Build history of the part. All positions in model axes, mm. Round coordinates to 2 decimals unless told otherwise and drop trailing zeros. Order: outer loops, then holes, each group sorted by start corner. A loop starts at its lowest first (then second) coordinate and runs counter-clockwise, first axis right, second up. Notation, with made-up numbers: (41.25, -24) -> (96.25, -24) arc R23 ccw to (96.25, 11) -> close; hole circle Ø8 at (40.25, -3). An arc over 180 degrees is marked (long way). Write item = value, one per line.
from build123d import *

# Parameters (mm, degrees)
F0_R     = 1.806666
F0_R_2   = 1.778
F0_R_3   = 6.35
F1_DEPTH = 6.35


with BuildPart() as f1:
    # F0 (on Front) → F1 (new body)
    with BuildSketch(Plane.XZ):
        Polygon((10.647724, 12.7), (-12.7, 12.7), (-12.7, -12.7), (10.647724, -12.7), (10.886472, -12.7), (10.886472, 12.7), align=None)
        with Locations((-6.35, -6.35)):
            Circle(F0_R, mode=Mode.SUBTRACT)
        with Locations((0, -8.825461)):
            Circle(F0_R_2, mode=Mode.SUBTRACT)
        with Locations((6.562257, -6.562257)):
            Circle(F0_R_2, mode=Mode.SUBTRACT)
        Circle(F0_R_3, mode=Mode.SUBTRACT)
        with Locations((8.869724, 0)):
            Circle(F0_R_2, mode=Mode.SUBTRACT)
        with Locations((-6.35, 6.35)):
            Circle(F0_R_2, mode=Mode.SUBTRACT)
        with Locations((6.35, 6.35)):
            Circle(F0_R_2, mode=Mode.SUBTRACT)
        with Locations((0, 8.742251)):
            Circle(F0_R_2, mode=Mode.SUBTRACT)
    extrude(amount=F1_DEPTH)


solid = f1.part
Q1. Cut at A-A, the plane z = 0. List the corners of the cut face in (x, y).
Check values:
outline = (-12.7, -6.35) -> (-6.35, -6.35) -> (-6.35, 0) -> (-12.7, 0) -> close; (6.35, -6.35) -> (7.09, -6.35) -> (7.09, 0) -> (6.35, 0) -> close; (10.65, -6.35) -> (10.89, -6.35) -> (10.89, 0) -> (10.65, 0) -> close
Q2. Cut at C-C, the plane x = -6. List the corners of the cut face in (y, z).
Check values:
outline = (-6.35, -12.7) -> (0, -12.7) -> (0, -8.12) -> (-6.35, -8.12) -> close; (-6.35, -4.58) -> (0, -4.58) -> (0, -2.08) -> (-6.35, -2.08) -> close; (-6.35, 2.08) -> (0, 2.08) -> (0, 4.61) -> (-6.35, 4.61) -> close; (-6.35, 8.09) -> (0, 8.09) -> (0, 12.7) -> (-6.35, 12.7) -> close
Q3. Cut at B-B, the plane x = 6.75. List the corners of the cut face in (y, z).
Check values:
outline = (-6.35, -12.7) -> (0, -12.7) -> (0, -8.33) -> (-6.35, -8.33) -> close; (-6.35, -4.79) -> (0, -4.79) -> (0, 4.62) -> (-6.35, 4.62) -> close; (-6.35, 8.08) -> (0, 8.08) -> (0, 12.7) -> (-6.35, 12.7) -> close
Q4. Mould opens along X. For faces 1 (the face through (-7.68, -3.13, -5.13)), 2 (the face through (-1, -3, -12.7)), 3 (the face through (-12.7, -3, 0)) say: released by +X, released by -X, zero draft, split by the parting line, or undercut.
Check values:
face_1 = undercut
face_2 = zero draft
face_3 = released by -X
Q5. Cut at D-D, the plane y = -5.5. Give the number of separate pieces and of enclosed holes in the cut face, and give its area (3 significant figures).
Check values:
separate_pieces = 1
enclosed_holes = 8
area = 403 mm²
Q6. Probe probe 1 along X at (y, z) = (-2.5, -6.5); probe 2 along Z at (x, y) = (0, -5); probe 3 along Z at (x, y) = (5, -1). List the from-to ranges inside material, lowest first.
Check values:
probe_1 = -12.7 to -8.15, -4.55 to 4.79, 8.34 to 10.89
probe_2 = -12.7 to -10.6, -7.05 to -6.35, 6.35 to 6.96, 10.52 to 12.7
probe_3 = -12.7 to -7.41, -5.71 to -3.91, 3.91 to 5.19, 7.51 to 12.7
Q7. Flat gauge pin, fed straight in: pin 1 (3.5 mm diameter, centred on x = -6.35, z = -6.35, fed in from +Y). Where does the tip first touch, or does it go through?
Check values:
pin_1 = through
